Autodesk Inventor part; units mm, degrees
ref_plane "YZ Plane" through (0, 0, 0) normal (1, 0, 0) x (0, 1, 0)
ref_plane "XZ Plane" through (0, 0, 0) normal (0, 1, 0) x (-1, 0, 0)
ref_plane "XY Plane" through (0, 0, 0) normal (0, 0, 1) x (1, 0, 0)
sketch "Sketch1" plane through (0, 0, 0) normal (0, 0, 1) x (1, 0, 0)
  line L0 (30, -10) -> (-30, -10)
  line L1 (0, 30.1987) -> (0, -10) construction
  line L2 (-30, -10) -> (-30, 10)
  line L3 (-30, 10) -> (-10, 50)
  line L4 (-10, 50) -> (10, 50)
  line L5 (10, 50) -> (30, 10)
  line L6 (30, 10) -> (30, -10)
  circle A0 centre (0, 0) radius 2.6
  circle A1 centre (-20, 0) radius 2.6
  circle A2 centre (20, 0) radius 2.6
  circle A3 centre (0, 0) radius 2.6
  circle A4 centre (0, 20) radius 2.6
  circle A5 centre (0, 40) radius 2.6
  point P0 (0, 50)
  dimension "d2" = 20
  dimension "d3" = 20
  dimension "d4" = 60
  dimension "d5" = 60
  dimension "d6" = 5.2
  dimension "d8" = 10
  dimension "d11" = 20
  dimension "d14" = 20
  dimension "d19" = 20
extrude "Extrusion1" add sketch "Sketch1" along normal blind 4
properties part number "T joining plate"
The model under review builds one solid part; all positions refer to its coordinate system, in mm. Give positions to 0.01 mm unless a question says otherwise; leave off trailing zeros. Order: outer loops, then holes, each group sorted by start corner. A loop starts at its lowest first (then second) coordinate and runs counter-clockwise, first axis right, second up. Notation, with made-up numbers: (25.25, 68.5) - (67.25, 68.5) arc R25 cw to (67.25, 85.5) - close; hole circle Ø6 at (85.25, 62.5). An arc over 180 degrees is marked (long way). Use CSV: the item, a comma, the result in double quotes. Start each with the question number.
Q1. To check wall thickness, follow line 1 along Y through (x, z) = (0, 2.65); line 2 along X through (y, z) = (0.5, 1.3); line 3 along Y through (x, z) = (-20, 2.5). State the ranges of each line that lie inside material, in increasing order. Write a range as [from, to].
Q2. The part is to be moulded in two halves that separate along Y. For faces 1 (the flat face through (0, 50, 2)), 2 (the cylindrical face through (-0.338, -2.578, 1.972)), 3 (the flat face through (30, 0, 2)), 4 (the cylindrical face through (22.48, -0.78, 1.97)), say which applies: +Y half, -Y half, draft (parallel to the pull), parting line (faces both ways), or undercut.
Q3. We need section B-B, the plane y = 40. Write out the cut boundary in (x, z).
Q4. We need section A-A, the plane x = 0. Write out the cut boundary in (y, z).
Q5. We need section D-D, the plane x = -20. Write out the cut boundary in (y, z), and give its area (3 significant figures).
Q6. Clearance check with flat-ended pins moving along their axes: pin 1 Ø2 at (y, z) = (19.5, 1.5) entering from -X; pin 2 Ø4.5 at (x, y) = (0, 40) entering from +Z; pin 3 Ø2 at (y, z) = (17.5, 1.5) entering from -X. State where each tip first meets the part, or that it passes through.
Q7. We need section C-C, the plane z = 0.6. Write out the cut boundary in (x, y).
Outcome:
1,line 1,"y = [-10, -2.6], [2.6, 17.4], [22.6, 37.4], [42.6, 50]"
1,line 2,"x = [-30, -22.55], [-17.45, -2.55], [2.55, 17.45], [22.55, 30]"
1,line 3,"y = [-10, -2.6], [2.6, 30]"
2,face 1,"+Y half"
2,face 2,"undercut"
2,face 3,"draft"
2,face 4,"undercut"
3,outline,"(-15, 0) - (-2.6, 0) - (-2.6, 4) - (-15, 4) - close; (2.6, 0) - (15, 0) - (15, 4) - (2.6, 4) - close"
4,outline,"(-10, 0) - (-2.6, 0) - (-2.6, 4) - (-10, 4) - close; (2.6, 0) - (17.4, 0) - (17.4, 4) - (2.6, 4) - close; (22.6, 0) - (37.4, 0) - (37.4, 4) - (22.6, 4) - close; (42.6, 0) - (50, 0) - (50, 4) - (42.6, 4) - close"
5,outline,"(-10, 0) - (-2.6, 0) - (-2.6, 4) - (-10, 4) - close; (2.6, 0) - (30, 0) - (30, 4) - (2.6, 4) - close"
5,area,"139 mm^2"
6,pin 1,"stops at x = -25.75"
6,pin 2,"passes through"
6,pin 3,"stops at x = -26.75"
7,outline,"(-30, -10) - (30, -10) - (30, 10) - (10, 50) - (-10, 50) - (-30, 10) - close; hole circle Ø5.2 at (-20, 0); hole circle Ø5.2 at (0, 0); hole circle Ø5.2 at (0, 20); hole circle Ø5.2 at (0, 40); hole circle Ø5.2 at (20, 0)"
